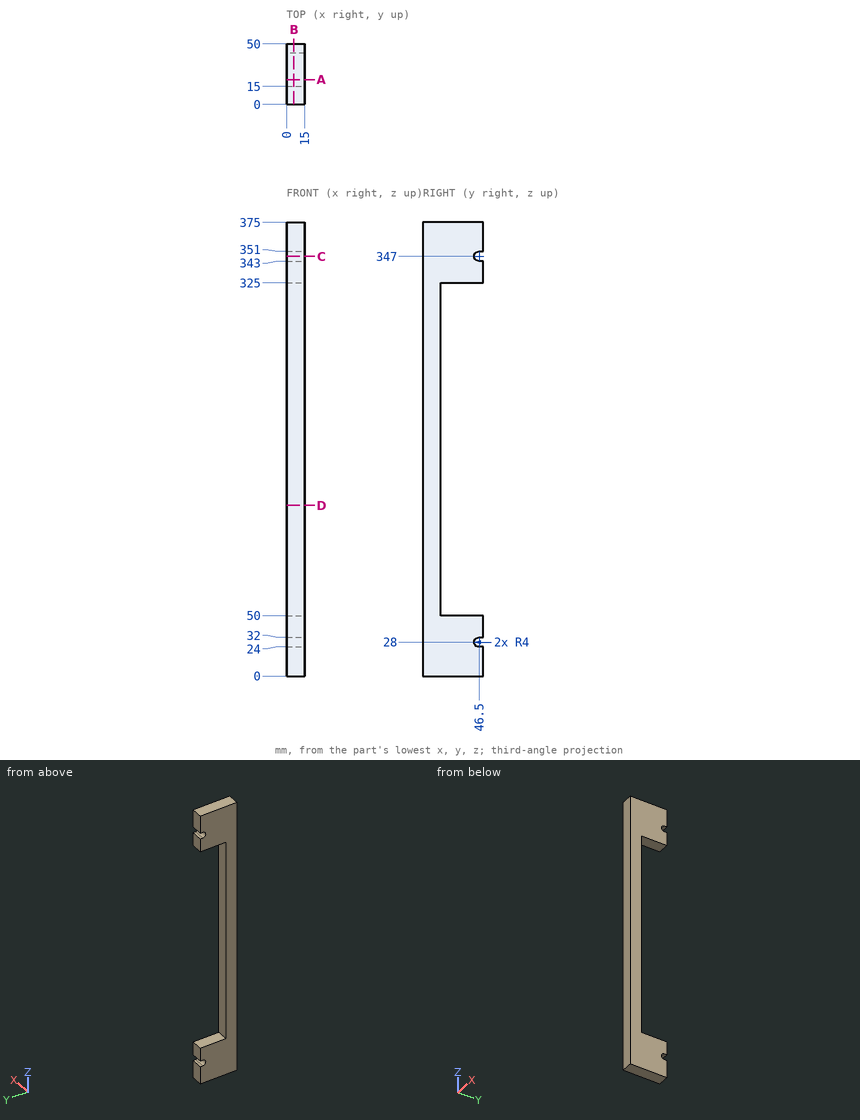
Here's the drawing with two shaded views (mm, measured from the low corner). I have some questions. Coordinates: 2 decimals unless noted, no trailing zeros. Write each loop counter-clockwise with the first axis right and the second up, starting at its lowest first coordinate (ties: lowest second). Pieces come first, ordered by that corner, then holes.
Item 1: I want a section at A-A on y = 20.5. Write out the boundary of the cut face in (x, z).
Item 2: If I drill on line 1 (Z direction, x = 1.5, y = 46.5); line 2 (Z direction, x = 8.25, y = 18.5); line 3 (Z direction, x = 10.75, y = 44), over which ranges is the centre line in solid material (lowest first)?
Item 3: I want a section at D-D on z = 141. Write out the boundary of the cut face in (x, y), and give its area (3 significant figures).
Item 4: I want a section at C-C on z = 347. Write out the boundary of the cut face in (x, y), and give its area (4 significant figures).
Item 5: I want a section at B-B on x = 6. Write out the boundary of the cut face in (y, z).
Findings below:
1. outline: (0, 0) - (15, 0) - (15, 50) - (0, 50) - close; (0, 325) - (15, 325) - (15, 375) - (0, 375) - close
2. line 1: z = 0 to 24, 32 to 50, 325 to 343, 351 to 375
2. line 2: z = 0 to 50, 325 to 375
2. line 3: z = 0 to 24.88, 31.12 to 50, 325 to 343.88, 350.12 to 375
3. outline: (0, 0) - (15, 0) - (15, 15) - (0, 15) - close
3. area: 225 mm2
4. outline: (0, 0) - (15, 0) - (15, 42.5) - (0, 42.5) - close
4. area: 637.5 mm2
5. outline: (0, 0) - (50, 0) - (50, 24) - (46.5, 24) arc R4 cw to (46.5, 32) - (50, 32) - (50, 50) - (15, 50) - (15, 325) - (50, 325) - (50, 343) - (46.5, 343) arc R4 cw to (46.5, 351) - (50, 351) - (50, 375) - (0, 375) - close
